Can you work these out from the model? Positions are in its coordinate system, mm. Face numbers are marked on the shaded views. A direction names the side the tool comes from. Round coordinates to 2 decimals unless told otherwise and drop trailing zeros. Order: outer loops, then holes, each group sorted by start corner. A loop starts at its lowest first (then second) coordinate and runs counter-clockwise, first axis right, second up.
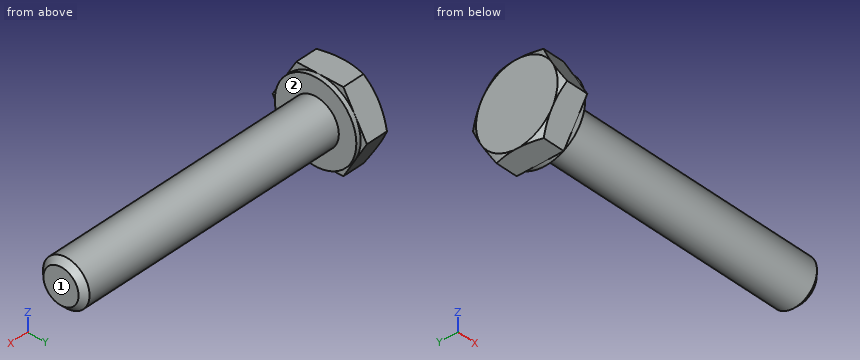
Autodesk Inventor part; units mm, degrees
ref_plane "Work Plane1" through (1.525, 0, 0) normal (0, 0, 1) x (1, 0, 0)
ref_plane "YZ Plane" through (0, 0, 0) normal (1, 0, 0) x (0, 1, 0)
ref_plane "XZ Plane" through (0, 0, 0) normal (0, 1, 0) x (-1, 0, 0)
sketch "Sketch1" plane through (0, 0, 0) normal (0, 0, 1) x (1, 0, 0)
  line L0 (0, 5.5626) -> (0, 3.175)
  line L1 (19.05, 3.175) -> (38.1, 3.175)
  line L2 (38.1, 3.175) -> (38.1, 0)
  line L3 (38.1, 0) -> (-0.6351, 0)
  line L4 (-8.3821, 0) -> (45.847, 0)
  line L5 (-0.6351, 0) -> (-0.6351, 5.5626)
  line L6 (-0.6351, 5.5626) -> (0, 5.5626)
  line L7 (19.05, 3.175) -> (8.8899, 3.175)
  line L8 (8.8899, 3.175) -> (0, 3.175)
  line L9 (0, -1.1125) -> (0, 6.6751)
  dimension "d0" = 38.1
  dimension "d1" = 19.05
  dimension "d2" = 6.35
  dimension "d9" = 0.6351
  dimension "d10" = 11.1252
  dimension "d13" = 10.1601
  dimension "d14" = 6.35
revolve "Body" add sketch "Sketch1" angle 360 about axis through (38.1, 0, 0) along (-1, 0, 0)
sketch "Sketch2" plane through (-0.6351, 0, 0) normal (-1, 0, 0) x (0, 0, 1)
  line L0 (0, 6.4231) -> (5.5626, 3.2116)
  line L1 (5.5626, 3.2116) -> (5.5626, -3.2116)
  line L2 (5.5626, -3.2116) -> (0, -6.4231)
  line L3 (0, -6.4231) -> (-5.5626, -3.2116)
  line L4 (-5.5626, -3.2116) -> (-5.5626, 3.2116)
  line L5 (-5.5626, 3.2116) -> (0, 6.4231)
  point P0 (0, 0)
  point P1 (0, 0)
  dimension "d11" = 11.1252
extrude "Head" add sketch "Sketch2" along normal blind 3.5052
sketch "Sketch4" plane through (0, 0, 0) normal (0, 0, 1) x (1, 0, 0)
  line L0 (-4.1403, 5.5626) -> (-4.1403, 6.4231)
  line L1 (-4.1403, 6.4231) -> (-3.6435, 6.4231)
  line L2 (-3.6435, 6.4231) -> (-4.1403, 5.5626)
  line L3 (-4.8413, 0) -> (0.0659, 0)
  line L4 (-0.6351, 6.4231) -> (-4.1403, 6.4231)
  line L5 (-4.1403, 3.2116) -> (-4.1403, 6.4231)
  dimension "d5" = 30
  dimension "d19" = 11.1252
revolve "Chamfer1" cut sketch "Sketch4" angle 360 about axis through (-10, 0, 0) along (1, 0, 0)
thread "Thread"
chamfer "Chamfer2" distance 0.779 distance2 0.7791 1 edges at (38.1, -3.175, 0) measured on face at (38.1, -0.7017, 0.0433)
ref_plane "Work Plane1" through (1.525, 0, 0) normal (0, 0, 1) x (1, 0, 0)
equation "\"d0\" = NLG"
equation "\"d1\" = GEL"
equation "\"d2\" = GD"
equation "\"d10\" = SD2"
equation "\"d14\" = BDM"
equation "\"d11\" = SW"
equation "\"d3\" = KOH - SD"
equation "\"d5\" = ANG1"
equation "\"d19\" = SW0"
equation "\"d15\" = GEL"
equation "\"d6\" = -0.5 * SPD + 0.5 * GD"
equation "\"NLG\" = 38.1"
equation "\"GD\" = 6.35"
equation "\"BDM\" = 6.35"
equation "\"KOH\" = 4.1402"
equation "\"GEL\" = 19.05"
equation "\"SW\" = 11.1252"
equation "\"SW0\" = SW"
equation "\"SPD\" = GD1"
equation "\"SD2\" = SW"
equation "\"SD\" = 0.635"
equation "\"ANG1\" = 30deg"
equation "\"GAL\" = 10.16"
equation "\"GUL\" = 0.77902"
equation "\"RR\" = 0.381"
equation "\"WFT\" = SD"
equation "\"GD1\" = 4.79196"
equation "\"THREADDIA\" = 6.35"
equation "\"SDH\" = SW"
equation "\"SDHG\" = 8.89"
equation "\"TOA\" = 30deg"
equation "\"FAWI\" = 45deg"
equation "\"NND\" = 6.35"
equation "\"E0\" = 12.84961"
properties part number "AS 2465 - 1/4 x 1 1/2  UNC" material "Steel, Mild"
(1) I want a section at A-A, the plane x = 1. List the corners of the cut face in (y, z) for me (3 decimals).
(2) On a 3-axis mill with a long thin cutter (end or side, diameter ignored), from which of +Z, -Z, +X, -X, +Y, -Y can I reach the whole of each face in a straight line? I mean the marked faces 1 and 2. Say none if no direction works.
(3) Please list where these lines run through material, in increasing order: probe 1 along X at (y, z) = (-2, 4.75); probe 2 along Z at (x, y) = (-0.5, -0.25); probe 3 along Y at (x, z) = (27, -1.5).
(4) I'm going to push flat-ended pins straight in: pin 1 Ø2 at (y, z) = (-3.5, 4) entering from +X; pin 2 Ø6 at (x, z) = (33, 0.5) entering from -Y (3 decimals); pin 3 Ø4 at (x, y) = (31, -3) entering from +Z. Where does each tip first touch, or does it pass through?
Ans:
1. outline: circle Ø6.35 at (0, 0)
2. face 1: +Z, -Z, +X, +Y, -Y
2. face 2: +X
3. probe 1: x = -4.14 to 0
3. probe 2: z = -5.56 to 5.56
3. probe 3: y = -2.8 to 2.8
4. pin 1: stops at x = 0
4. pin 2: stops at y = -3.175
4. pin 3: stops at z = 3.01
